Input: part model. Units: mm. Frame: model coordinates. A direction names the side the tool comes from. Round coordinates to 2 decimals unless told otherwise and drop trailing zeros. Order: outer loops, then holes, each group sorted by start corner. A loop starts at its lowest first (then second) coordinate and runs counter-clockwise, first axis right, second up. Notation, with made-up numbers: M 69,33 L 91,33 A18 cw 91,48 Z; hole C 20,17 d6. An arc over 180 degrees is marked long. One line per question, with ' | ' between items.
Autodesk Inventor part; units mm, degrees
ref_plane "YZ Plane" through (0, 0, 0) normal (1, 0, 0) x (0, 1, 0)
ref_plane "XZ Plane" through (0, 0, 0) normal (0, 1, 0) x (-1, 0, 0)
ref_plane "XY Plane" through (0, 0, 0) normal (0, 0, 1) x (1, 0, 0)
sketch "Sketch1" plane through (0, 0, 0) normal (0, 0, 1) x (1, 0, 0)
  line L0 (-290, -30) -> (290, -30)
  line L1 (290, -30) -> (290, 30)
  line L2 (290, 30) -> (-290, 30)
  line L3 (-290, 30) -> (-290, -30)
  line L4 (-290, -30) -> (290, 30) construction
  line L5 (290, -30) -> (-290, 30) construction
  line L6 (-290, 9.925) -> (-294.9, 9.925)
  line L7 (-294.9, 9.925) -> (-294.9, -9.925)
  line L8 (-294.9, -9.925) -> (-290, -9.925)
  line L9 (-290, -9.925) -> (-290, 9.925)
  line L10 (0, 30) -> (0, -30)
  line L11 (290, 9.925) -> (294.9, 9.925)
  line L12 (294.9, 9.925) -> (294.9, -9.925)
  line L13 (294.9, -9.925) -> (290, -9.925)
  line L14 (290, -9.925) -> (290, 9.925)
  point P0 (0, 0)
  point P1 (-290, 0)
  point P2 (-290, 0)
  point P3 (290, 0)
  point P4 (290, 0)
  dimension "d0" = 580
  dimension "d1" = 60
  dimension "d2" = 4.9
  dimension "d3" = 19.85
extrude "Plate1" add sketch "Sketch1" along normal blind 5
sketch "Sketch2" plane through (0, 0, 5) normal (0, 0, 1) x (1, 0, 0)
  line L0 (-230, 0) -> (-80, 0) construction
  line L1 (-230, -12) -> (-80, -12)
  line L2 (-80, 12) -> (-230, 12)
  arc A0 (-230, 12) -> (-230, -12) centre (-230, 0) ccw
  arc A1 (-80, -12) -> (-80, 12) centre (-80, 0) ccw
  line L3 (0, 30) -> (0, -30)
  line L4 (290, -30) -> (-290, -30)
  line L5 (-290, 30) -> (290, 30)
  line L6 (230, 0) -> (80, 0) construction
  line L7 (230, -12) -> (80, -12)
  line L8 (80, 12) -> (230, 12)
  arc A2 (230, -12) -> (230, 12) centre (230, 0) ccw
  arc A3 (80, 12) -> (80, -12) centre (80, 0) ccw
  point P0 (0, 0)
  point P1 (-155, 0)
  point P2 (155, 0)
  dimension "d5" = 12
  dimension "d6" = 150
  dimension "d7" = 80
extrude "Cut1" cut sketch "Sketch2" against normal blind 5
equation "\"d8\" = Thickness"
equation "\"d4\" = Thickness"
equation "\"BendRadius\" = Thickness"
equation "\"BendReliefWidth\" = Thickness"
equation "\"BendReliefDepth\" = 0.5 * Thickness"
equation "\"TransitionRadius\" = BendRadius"
equation "\"JacobiRadiusSize\" = BendRadius"
equation "\"GapSize\" = Thickness"
properties part number "Table-Base Supporter 1st"
Item 1: Section query B-B, the plane x = -182.5. Return loops of the section in (y, z), plus the area to 3 significant figures.
Report:
outline: M -30,0 L -12,0 L -12,5 L -30,5 Z; M 12,0 L 30,0 L 30,5 L 12,5 Z | area: 180 mm²
Item 2: Access query for faces 4 (the flat face through (-4, 0, 0)), 5 (the cylindrical face through (-242, 0, 3)). Directions: +Z, -Z, +X, -X, +Y, -Y. A direction counts if a zero-diameter tool reaches every point of the face in a straight line with its end or side. Return the directions, or none.
Report:
face 4: -Z, +X, -X, +Y, -Y | face 5: +Z, -Z
Item 3: Line query: line 1 along X through (y, z) = (1, 4.7); line 2 along Y through (x, z) = (115, 3.05); line 3 along X through (y, z) = (6.5, 1.3). Output: solid intervals per line, ascending. Write a range as from..to.
Report:
line 1: -294.9..-241.96, -68.04..68.04, 241.96..294.9 | line 2: -30..-12, 12..30 | line 3: -294.9..-240.09, -69.91..69.91, 240.09..294.9
Item 4: Section query C-C, the plane y = -18. Return loops of the section in (x, z), plus the area to 3 significant figures.
Report:
outline: M -290,0 L 290,0 L 290,5 L -290,5 Z | area: 2,900 mm²
Item 5: First-contact query: pin 1 (1.5 mm diameter, centred on y = 16, z = 2.5, fed in from +X); pin 2 (12 mm diameter, centred on x = -78, y = -2, fed in from -Z); pin 3 (1.5 mm diameter, centred on x = 292, z = 3.5, fed in from -Y) (3 decimals); pin 4 (2.5 mm diameter, centred on y = 21, z = 2, fed in from -X). Flat tips, straight axial feed; report the tip coordinate or a pass-through.
Report:
pin 1: x = 290 | pin 2: through | pin 3: y = -9.925 | pin 4: x = -290
Item 6: Section query A-A, the plane z = 2.7. Return loops of the section in (x, y) (3 decimals).
Report:
outline: M -294.9,-9.925 L -290,-9.925 L -290,-30 L 290,-30 L 290,-9.925 L 294.9,-9.925 L 294.9,9.925 L 290,9.925 L 290,30 L -290,30 L -290,9.925 L -294.9,9.925 Z; hole M -230,-12 L -80,-12 A12 ccw -80,12 L -230,12 A12 ccw Z; hole M 80,-12 L 230,-12 A12 ccw 230,12 L 80,12 A12 ccw Z
Item 7: Mould query, pull axis Y, two halves, no side actions, for faces 1 (the cylindrical face through (242, 0, 3)), 2 (the flat face through (-4, 0, 5)), 3 (the cylindrical face through (-68, 0, 3)). Classes: +Y half, -Y half, draft (parallel to the pull), parting line (faces both ways), or undercut.
Report:
face 1: undercut | face 2: draft | face 3: undercut
